```python
from build123d import *

# Parameters (mm, degrees)
SKETCH_R   = 0.4
SKETCH_R_2 = 0.3
SKETCH_R_3 = 0.2
PAD_DEPTH  = 3


with BuildPart() as part:
    # Sketch → Pad (new body)
    with BuildSketch(Plane.XY):
        Polygon((0, 0), (9, 0), (9, 9), (0, 9), (0, 7), (0, 4.5), (0, 2), align=None)
        with Locations((2, 2)):
            Circle(SKETCH_R, mode=Mode.SUBTRACT)
        with Locations((4.5, 2)):
            Circle(SKETCH_R_2, mode=Mode.SUBTRACT)
        with Locations((7, 2)):
            Circle(SKETCH_R_3, mode=Mode.SUBTRACT)
        with Locations((2, 4.5)):
            Circle(SKETCH_R, mode=Mode.SUBTRACT)
        with Locations((4.5, 4.5)):
            Circle(SKETCH_R_2, mode=Mode.SUBTRACT)
        with Locations((7, 4.5)):
            Circle(SKETCH_R_3, mode=Mode.SUBTRACT)
        with Locations((2, 7)):
            Circle(SKETCH_R, mode=Mode.SUBTRACT)
        with Locations((4.5, 7)):
            Circle(SKETCH_R_2, mode=Mode.SUBTRACT)
        with Locations((7, 7)):
            Circle(SKETCH_R_3, mode=Mode.SUBTRACT)
    extrude(amount=PAD_DEPTH)


solid = part.part
```
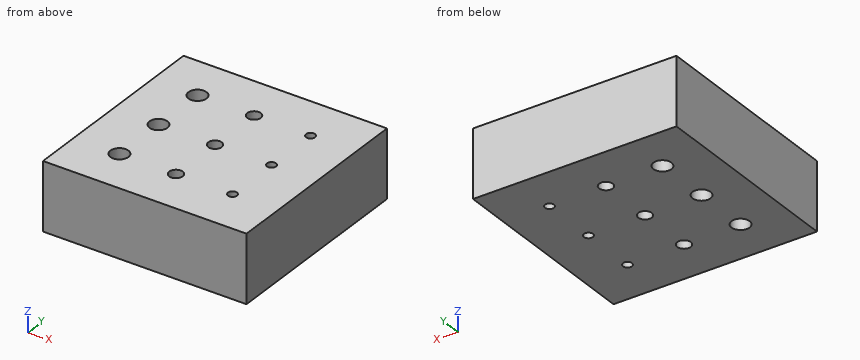
CAD build for the part. Positions are in the model's coordinates, mm. Round coordinates to 2 decimals unless told otherwise and drop trailing zeros. Loops run counter-clockwise (first coordinate to the right, second up) from the corner with the lowest first, then second, coordinate; pieces in that order, holes last. Notation, with made-up numbers: M -6,-12 L 53,-12 A24 cw 53,19 Z; hole C -9,86 d6. An arc over 180 degrees is marked long. Return JSON: item names as keys, results as strings. Group by question number.
(1) Saw through at C-C, the plane z = 0.7. Give the number of separate pieces and of enclosed holes in the cut face, and give its area (3 significant figures).
(2) Wall check: probe 1 along Y at (x, z) = (4.5, 2.25); probe 2 along Y at (x, z) = (2, 2.2). Give the ranges that are in metal, low to high. Write a range as [from, to].
(3) Saw through at B-B, the plane y = 2. List the corners of the cut face in (x, z).
(4) Saw through at A-A, the plane x = 2. List the corners of the cut face in (y, z).
Answer list:
{
 "1": {"separate pieces": "1", "enclosed holes": "9", "area": "78.3 mm2"},
 "2": {"probe 1": "[0, 1.7], [2.3, 4.2], [4.8, 6.7], [7.3, 9]", "probe 2": "[0, 1.6], [2.4, 4.1], [4.9, 6.6], [7.4, 9]"},
 "3": {"outline": "M 0,0 L 1.6,0 L 1.6,3 L 0,3 Z; M 2.4,0 L 4.2,0 L 4.2,3 L 2.4,3 Z; M 4.8,0 L 6.8,0 L 6.8,3 L 4.8,3 Z; M 7.2,0 L 9,0 L 9,3 L 7.2,3 Z"},
 "4": {"outline": "M 0,0 L 1.6,0 L 1.6,3 L 0,3 Z; M 2.4,0 L 4.1,0 L 4.1,3 L 2.4,3 Z; M 4.9,0 L 6.6,0 L 6.6,3 L 4.9,3 Z; M 7.4,0 L 9,0 L 9,3 L 7.4,3 Z"}
}
